Here's how the part is built. I have some questions about the finished solid (model axes, mm). Face numbers are marked on the shaded views. A direction names the side the tool comes from. Coordinates: 2 decimals unless noted, no trailing zeros. Write each loop counter-clockwise with the first axis right and the second up, starting at its lowest first coordinate (ties: lowest second). Pieces come first, ordered by that corner, then holes. Notation, with made-up numbers: (-4, 52) -> (18, 52) arc R36 ccw to (18, 87) -> close; hole circle Ø3 at (-36, 50.5). An arc over 180 degrees is marked (long way). Put each result on its own line as item: value.
```python
from build123d import *

# Parameters (mm, degrees)
F1_DEPTH = 71.12
F2_DEPTH = 2.54
F0_W     = 8.9689344168
F0_H     = 4.2472973967
F3_DEPTH = 82.042


with BuildPart() as f1:
    # F0 (on Top) → F1 (new body)
    with BuildSketch(Plane.XY):
        Polygon((39.6875, -31.115), (39.6875, 31.115), (8.9689344168, 31.115), (8.9689344168, 26.8677026033), (35.836905241, 26.8677026033), (35.836905241, -26.8677026033), (0, -26.8677026033), (0, -31.115), align=None)
        Polygon((-39.6875, -31.115), (0, -31.115), (0, -26.8677026033), (-35.836905241, -26.8677026033), (-35.836905241, 26.8677026033), (-8.9689344168, 26.8677026033), (-8.9689344168, 31.115), (-39.6875, 31.115), align=None)
    extrude(amount=F1_DEPTH)

    # F0 (on Top) → F2 (join)
    with BuildSketch(Plane.XY):
        Polygon((35.836905241, 26.8677026033), (8.9689344168, 26.8677026033), (0, 26.8677026033), (0, -26.8677026033), (35.836905241, -26.8677026033), align=None)
        Polygon((0, -26.8677026033), (0, 26.8677026033), (-8.9689344168, 26.8677026033), (-35.836905241, 26.8677026033), (-35.836905241, -26.8677026033), align=None)
    extrude(amount=F2_DEPTH)

    # F0 (on Top) → F3 (join)
    with BuildSketch(Plane.XY):
        with Locations((-4.4844672084, 28.9913513017)):
            Rectangle(F0_W, F0_H)
        with Locations((4.4844672084, 28.9913513017)):
            Rectangle(F0_W, F0_H)
    extrude(amount=F3_DEPTH)


solid = f1.part
```
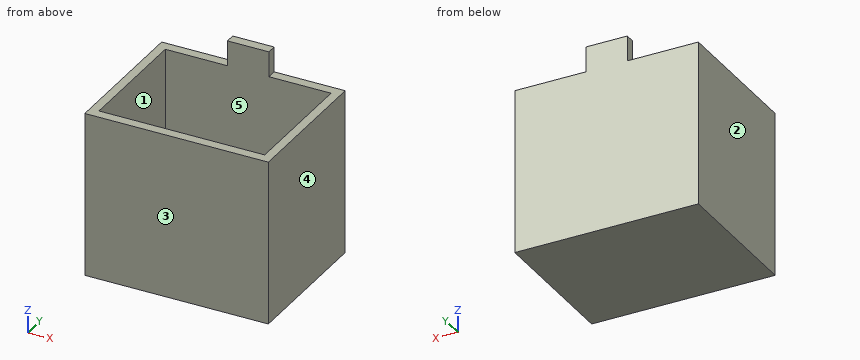
Item 1: Please list where these lines run through material, in increasing order: line 1 along Y through (x, z) = (11.5, 45.5) (3 decimals); line 2 along X through (y, z) = (19.5, 68.5); line 3 along Z through (x, y) = (-9, 19). Write a range as from..to.
Output:
line 1: y = -31.115..-26.868, 26.868..31.115
line 2: x = -39.69..-35.84, 35.84..39.69
line 3: z = 0..2.54
Item 2: For P1, Ø2, axis at y = 28, z = 79, coming from the +X side; P2, Ø1.3, axis at y = 28.5, z = 77.5, coming from the -X side; P3, Ø18.5, axis at x = -10, y = -11.5, coming from the +Z side, each with a flat end and sliding along its axis, tell me the tip position at first contact or that it passes through.
Output:
P1: stops at x = 8.97
P2: stops at x = -8.97
P3: stops at z = 2.54
Item 3: Imagine slicing it at D-D on z = 76.5. Write out the boundary of the cut face in (x, y) (3 decimals).
Output:
outline: (-8.969, 26.868) -> (8.969, 26.868) -> (8.969, 31.115) -> (-8.969, 31.115) -> close
Item 4: Imagine slicing it at B-B on x = -26. Write out the boundary of the cut face in (y, z) (3 decimals).
Output:
outline: (-31.115, 0) -> (31.115, 0) -> (31.115, 71.12) -> (26.868, 71.12) -> (26.868, 2.54) -> (-26.868, 2.54) -> (-26.868, 71.12) -> (-31.115, 71.12) -> close
Item 5: Imagine slicing it at A-A on z = 40.5. Write out the boundary of the cut face in (x, y) (1 decimal).
Output:
outline: (-39.7, -31.1) -> (39.7, -31.1) -> (39.7, 31.1) -> (-39.7, 31.1) -> close; hole (-35.8, -26.9) -> (35.8, -26.9) -> (35.8, 26.9) -> (-35.8, 26.9) -> close
Item 6: Imagine slicing it at C-C on y = -4. Write out the boundary of the cut face in (x, z).
Output:
outline: (-39.69, 0) -> (39.69, 0) -> (39.69, 71.12) -> (35.84, 71.12) -> (35.84, 2.54) -> (-35.84, 2.54) -> (-35.84, 71.12) -> (-39.69, 71.12) -> close
Item 7: If we mould it in two halves opening along Y, with no side actions, what happens to the marked faces 1, 2 and 3? For each: released by +Y, released by -Y, zero draft, split by the parting line, or undercut.
Output:
face 1: undercut
face 2: zero draft
face 3: released by -Y
Item 8: Which directions (+Z, -Z, +X, -X, +Y, -Y) give clear straight access to the entire face, cutting with the end or side of a thin tool? Please do the marked faces 4 and 5.
Output:
face 4: +Z, -Z, +X, +Y, -Y
face 5: +Z
